Read the model definition and answer for the solid it produces. Units are mm, in the model's axes. Give positions to 0.01 mm unless a question says otherwise; leave off trailing zeros. Write each question's results on one line, items separated by ' | '. Start each with the question number.
Q1. Flat-ended cylindrical pins translate along their axes: P1, Ø4.5, axis at y = -1.5, z = 205, coming from the +X side; P2, Ø1.5, axis at x = 3.5, z = 48, coming from the +Y side; P3, Ø2.5, axis at y = 1, z = 148.5, coming from the -X side. Find the tip coordinate at first contact, or state that the pin passes through.
Q2. Find section A-A on z = 82.5. Count the separate pieces of the cut face and the enclosed holes in it, and give its area (3 significant figures).
Q3. Find the intervals of material crossed by line 1 along X through (y, z) = (15, 119); line 2 along Y through (x, z) = (16, 367); line 3 along Y through (x, z) = (-5, 360), in increasing order. Write a range as from..to.
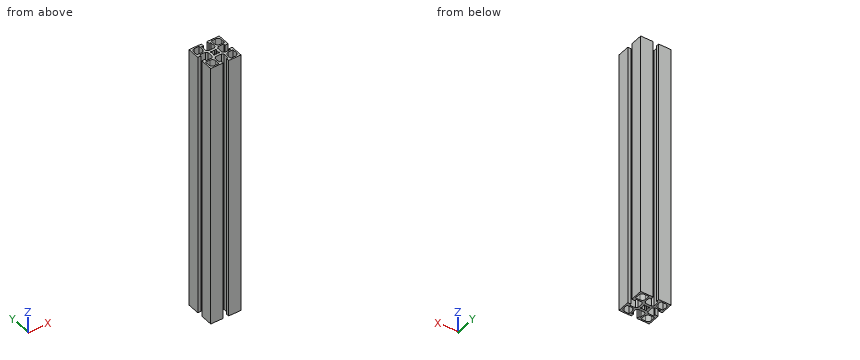
from build123d import *

# Parameters (mm, degrees)
BOSS_EXTRUDE1_DEPTH = 395


with BuildPart() as part:
    # Sketch1 → Boss-Extrude1 (new body)
    with BuildSketch(Plane.XY):
        Polygon((-17.999999991, -6.799999991), (-17.999999991, -4.099999991), (-22.499999991, -4.099999991), (-22.499999991, -22.499999991), (-4.099999991, -22.499999991), (-4.099999991, -17.999999991), (-6.799999991, -17.999999991), (-6.799999991, -9.499999991), (-4.499999991, -7.199999991), (4.500000009, -7.199999991), (6.800000009, -9.499999991), (6.800000009, -17.999999991), (4.100000009, -17.999999991), (4.100000009, -22.499999991), (22.500000009, -22.499999991), (22.500000009, -4.099999991), (18.000000009, -4.099999991), (18.000000009, -6.799999991), (9.500000009, -6.799999991), (7.200000009, -4.499999991), (7.200000009, 4.500000009), (9.500000009, 6.800000009), (18.000000009, 6.800000009), (18.000000009, 4.100000009), (22.500000009, 4.100000009), (22.500000009, 22.500000009), (4.100000009, 22.500000009), (4.100000009, 18.000000009), (6.800000009, 18.000000009), (6.800000009, 9.500000009), (4.500000009, 7.200000009), (-4.499999991, 7.200000009), (-6.799999991, 9.500000009), (-6.799999991, 18.000000009), (-4.099999991, 18.000000009), (-4.099999991, 22.500000009), (-22.499999991, 22.500000009), (-22.499999991, 4.100000009), (-17.999999991, 4.100000009), (-17.999999991, 6.800000009), (-9.499999991, 6.800000009), (-7.199999991, 4.500000009), (-7.199999991, -4.499999991), (-9.499999991, -6.799999991), align=None)
        with BuildLine():
            Line((-20.499999973, 8.799995438), (-20.499999973, 15.500000009))
            ThreePointArc((-20.499999973, 15.500000009), (-19.035533879, 19.035533915), (-15.499999973, 20.500000009))
            Line((-15.499999973, 20.500000009), (-8.799995402, 20.500000009))
            Line((-8.799995402, 20.500000009), (-8.799995402, 13.799995438))
            ThreePointArc((-8.799995402, 13.799995438), (-10.264461496, 10.264461532), (-13.799995402, 8.799995438))
            Line((-13.799995402, 8.799995438), (-20.499999973, 8.799995438))
        make_face(mode=Mode.SUBTRACT)
        with BuildLine():
            Line((20.500000009, 8.79999542), (13.799995438, 8.79999542))
            ThreePointArc((13.799995438, 8.79999542), (10.264461532, 10.264461514), (8.799995438, 13.79999542))
            Line((8.799995438, 13.79999542), (8.799995438, 20.499999991))
            Line((8.799995438, 20.499999991), (15.500000009, 20.499999991))
            ThreePointArc((15.500000009, 20.499999991), (19.035533915, 19.035533897), (20.500000009, 15.499999991))
            Line((20.500000009, 15.499999991), (20.500000009, 8.79999542))
        make_face(mode=Mode.SUBTRACT)
        with BuildLine():
            Line((15.499999991, -20.499999991), (8.79999542, -20.499999991))
            Line((8.79999542, -20.499999991), (8.79999542, -13.79999542))
            ThreePointArc((8.79999542, -13.79999542), (10.264461514, -10.264461514), (13.79999542, -8.79999542))
            Line((13.79999542, -8.79999542), (20.499999991, -8.79999542))
            Line((20.499999991, -8.79999542), (20.499999991, -15.499999991))
            ThreePointArc((20.499999991, -15.499999991), (19.035533897, -19.035533897), (15.499999991, -20.499999991))
        make_face(mode=Mode.SUBTRACT)
        with BuildLine():
            Line((-8.79999542, -20.499999973), (-15.499999991, -20.499999973))
            ThreePointArc((-15.499999991, -20.499999973), (-19.035533897, -19.035533879), (-20.499999991, -15.499999973))
            Line((-20.499999991, -15.499999973), (-20.499999991, -8.799995402))
            Line((-20.499999991, -8.799995402), (-13.79999542, -8.799995402))
            ThreePointArc((-13.79999542, -8.799995402), (-10.264461514, -10.264461496), (-8.79999542, -13.799995402))
            Line((-8.79999542, -13.799995402), (-8.79999542, -20.499999973))
        make_face(mode=Mode.SUBTRACT)
        with BuildLine():
            Line((-3.262737816, 1.848524254), (-4.596194076, 3.181980514))
            Line((-4.596194076, 3.181980514), (-3.181980513, 4.596194076))
            Line((-3.181980513, 4.596194076), (-1.848524253, 3.262737816))
            ThreePointArc((-1.848524253, 3.262737816), (2e-09, 3.749999997), (1.848524257, 3.262737816))
            Line((1.848524257, 3.262737816), (3.181980517, 4.596194076))
            Line((3.181980517, 4.596194076), (4.59619408, 3.181980513))
            Line((4.59619408, 3.181980513), (3.26273782, 1.848524253))
            ThreePointArc((3.26273782, 1.848524253), (3.75, -2e-09), (3.262737819, -1.848524257))
            Line((3.262737819, -1.848524257), (4.596194079, -3.181980517))
            Line((4.596194079, -3.181980517), (3.181980517, -4.596194079))
            Line((3.181980517, -4.596194079), (1.848524257, -3.262737819))
            ThreePointArc((1.848524257, -3.262737819), (2e-09, -3.75), (-1.848524253, -3.262737819))
            Line((-1.848524253, -3.262737819), (-3.181980515, -4.596194081))
            Line((-3.181980515, -4.596194081), (-4.596194078, -3.181980518))
            Line((-4.596194078, -3.181980518), (-3.262737816, -1.848524257))
            ThreePointArc((-3.262737816, -1.848524257), (-3.749999997, -2e-09), (-3.262737816, 1.848524254))
        make_face(mode=Mode.SUBTRACT)
    extrude(amount=BOSS_EXTRUDE1_DEPTH)


solid = part.part
Working result:
1) P1: x = 7.2 | P2: y = 22.5 | P3: x = -7.2
2) separate pieces: 1 | enclosed holes: 5 | area: 748 mm²
3) line 1: -22.5..-20.5, -8.8..-6.8, 6.8..8.8, 20.5..22.5 | line 2: -22.5..-20.47, -8.8..-6.8, 6.8..8.8, 20.47..22.5 | line 3: -22.5..-18, -7.7..7.7, 18..22.5
